Check sheet for the modelled part. Datum: model origin and axes. Units: mm. Face numbers are marked on the shaded views. A direction names the side the tool comes from. Give positions to 0.01 mm unless a question says otherwise; leave off trailing zeros. Loops run counter-clockwise (first coordinate to the right, second up) from the corner with the lowest first, then second, coordinate; pieces in that order, holes last. Notation, with made-up numbers: M 78,17.5 L 136,17.5 A37 ccw 136,56.5 Z; hole C -26,-7.5 d3. An arc over 180 degrees is marked long. Put each result on its own line as item: value. Start each with the question number.
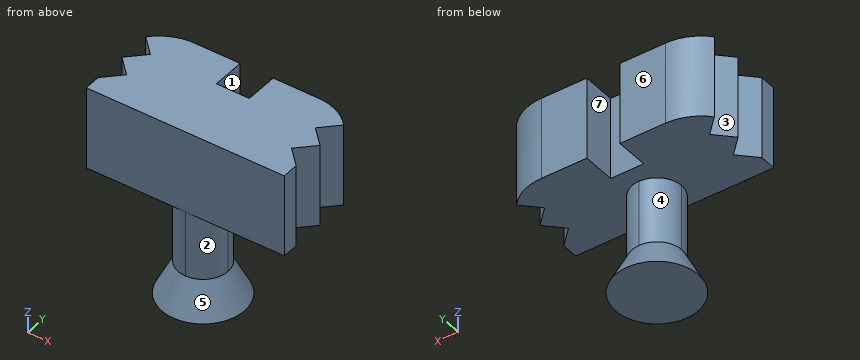
```python
from build123d import *

# Parameters (mm, degrees)
F0_W        = 2
F0_H        = 2
F1_DEPTH    = 5
F2_W        = 3
F2_H        = 3
F3_DEPTH    = 4
F4_R        = 1.49999
F5_W        = 2
F5_H        = 2
F6_DEPTH    = 5
F8_DEPTH    = 9.001
F9_T1_DEPTH = 16.1803398875
F10_R       = 1.5
F12_R       = 2.5


# Not quite as in the source:
# - a fillet or chamfer that OpenCascade refuses, or shapes differently, is made with other operations: its cross-section is extruded or revolved along the edge and cut away or added
# - a fillet or chamfer is up to 0.001 mm smaller than in the source, because OpenCascade refuses the exact size


with BuildPart() as f1:
    # F0 (on Top) → F1 (new body)
    with BuildSketch(Plane.XY):
        Polygon((-6, -3), (6, -3), (6, 3), (1, 3), (1, 1), (-1, 1), (-1, 3), (-6, 3), align=None)
        with Locations((0, 2)):
            Rectangle(F0_W, F0_H)
    extrude(amount=F1_DEPTH)

    # F2 (on face) → F3 (join)
    with BuildSketch(Plane(origin=(0, 0, 0), x_dir=(1, 0, 0), z_dir=(0, 0, -1))):
        with Locations((0, 1.5)):
            Rectangle(F2_W, F2_H)
    extrude(amount=F3_DEPTH)

    # F4 (radius 1.5 in the source; OpenCascade refuses exactly that, so slightly less here)
    f4_edges = [f1.edges().sort_by_distance(p)[0] for p in [
        (-1.5, 0, -2),
        (1.5, 0, -2),
        (-1.5, -3, -2),
        (1.5, -3, -2),
    ]]
    fillet(f4_edges, radius=F4_R)

    # F5 (on face) → F6 (cut, through all)
    with BuildSketch(Plane.XY.offset(5)):
        with Locations((0, 2)):
            Rectangle(F5_W, F5_H)
    extrude(amount=-F6_DEPTH, mode=Mode.SUBTRACT)

    # F7 (on face) → F8 (cut, through all)
    with BuildSketch(Plane.XY.offset(5)):
        Polygon((-5, 1), (-6, 2), (-6, 0), align=None)
        Polygon((-5, -1), (-6, 0), (-6, -2), align=None)
        Polygon((6, -2), (6, 0), (5, -1), align=None)
        Polygon((6, 0), (6, 2), (5, 1), align=None)
    extrude(amount=-F8_DEPTH, mode=Mode.SUBTRACT)

    # F9: fillet of radius 3 on 2 edges, made by hand

    # F9_s2 → F9_t1 (cut)
    with BuildSketch(Plane.XY.offset(-5.5901699437)):
        with BuildLine():
            ThreePointArc((-6, 2), (-4.9886768939, 2.7386127875), (-3.7639320225, 3))
            Line((-3.7639320225, 3), (-6, 3))
            Line((-6, 3), (-6, 2))
        make_face()
        with BuildLine():
            ThreePointArc((3.7639320225, 3), (4.9886768939, 2.7386127875), (6, 2))
            Line((6, 2), (6, 3))
            Line((6, 3), (3.7639320225, 3))
        make_face()
    extrude(amount=F9_T1_DEPTH, mode=Mode.SUBTRACT)

    # F10 (on face) → F13 section 0
    with BuildSketch(Plane(origin=(0, 0, -4), x_dir=(1, 0, 0), z_dir=(0, 0, -1))):
        with Locations((0, 1.5)):
            Circle(F10_R)
    # F12 (on offset) → F13 section 1
    with BuildSketch(Plane(origin=(0, 0, -6), x_dir=(1, 0, 0), z_dir=(0, 0, -1))):
        with Locations((0, 1.5)):
            Circle(F12_R)
    loft()


solid = f1.part
```
Q1. Section check B-B, the plane y = 1.75. Record the cut outline in (x, z), then the cut area to 3 significant figures.
Q2. Depth check by flat-ended pin: P1, Ø3, axis at x = 2, y = 1, coming from the -Z side; P2, Ø1, axis at x = 0, z = 2, coming from the +Y side; P3, Ø2.5, axis at x = 2, z = -1, coming from the -Y side. Enter the tip coordinate at first touch or a pass-through.
Q3. Thickness scan on line 1 along Y through (x, z) = (-3.5, 2); line 2 along Z through (x, y) = (-3, 1.25); line 3 along Z through (x, y) = (1.5, -0.25). Record the ranges inside material, lowest first. Write a range as [from, to].
Q4. Section check A-A, the plane z = 3.5. Record the cut outline in (x, y).
Q5. Mould release check, pull along X, two halves, no side actions. Record for the marked faces 5, 6 and 7: pulls with the +X half, pulls with the -X half, needs draft (parallel to the pull), parting line crosses it, or undercut.
Q6. Section check D-D, the plane x = 4. Record the cut outline in (y, z).
Q7. Access from +Z, -Z, +X, -X, +Y, -Y to the whole of each face (thin tool, end or side, straight path). Record for the marked faces 1, 2, 3 and 4.
Found:
1. outline: M -5.75,0 L -1,0 L -1,5 L -5.75,5 Z; M 1,0 L 5.75,0 L 5.75,5 L 1,5 Z
1. area: 47.5 mm^2
2. P1: stops at z = -6
2. P2: stops at y = 1
2. P3: stops at y = -3
3. line 1: y = [-3, 3]
3. line 2: z = [0, 5]
3. line 3: z = [-6, -4.91], [0, 5]
4. outline: M -6,-3 L 6,-3 L 6,-2 L 5,-1 L 6,0 L 5,1 L 6,2 A3 ccw 3.76,3 L 1,3 L 1,1 L -1,1 L -1,3 L -3.76,3 A3 ccw -6,2 L -5,1 L -6,0 L -5,-1 L -6,-2 Z
5. face 5: parting line crosses it
5. face 6: needs draft
5. face 7: undercut
6. outline: M -3,0 L 2.99,0 L 2.99,5 L -3,5 Z
7. face 1: +Z, -Z, +Y
7. face 2: +X, -Y
7. face 3: +Z, -Z, -X
7. face 4: -X, +Y
